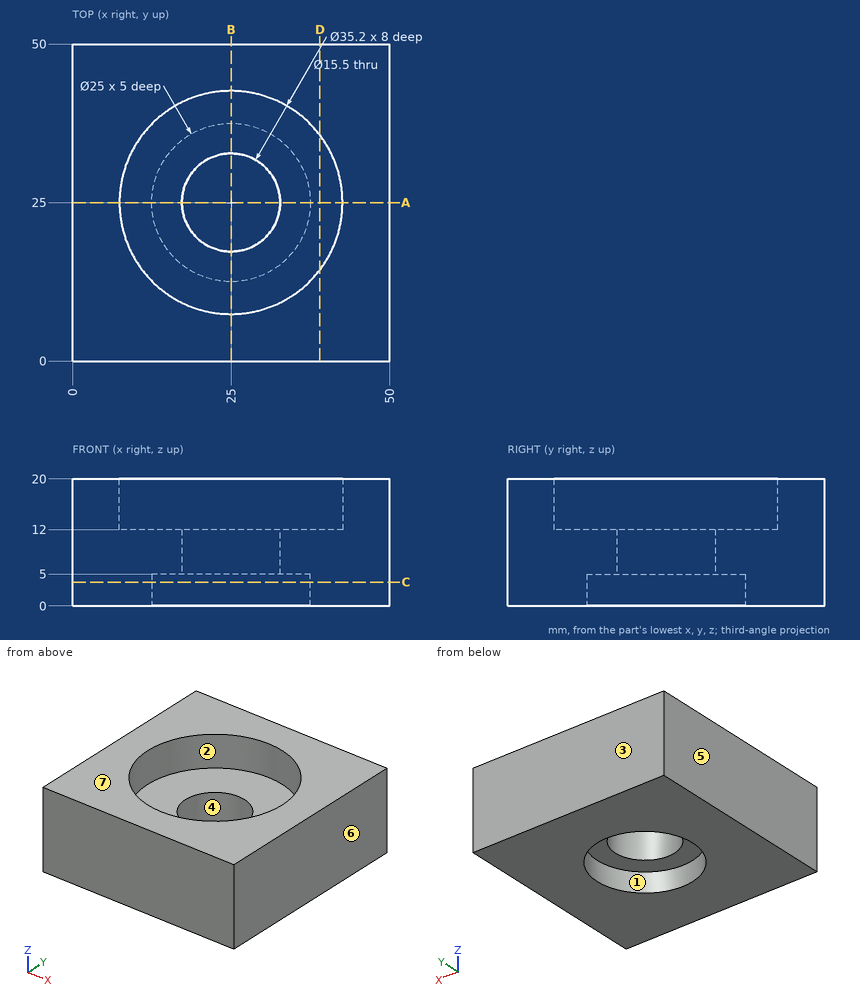
Answer from the drawing. Dimensions are ordinates in mm from the lowest x, y and z of the part. A direction names the side the tool comes from. Give positions to 0.01 mm unless a question says otherwise; leave off trailing zeros. Loops run counter-clockwise (first coordinate to the right, second up) from the corner with the lowest first, then second, coordinate; pieces in that order, holes last. Notation, with made-up numbers: (19, -30.5) -> (66, -30.5) arc R9 cw to (66, -22.5) -> close; hole circle Ø10 at (21, 6.5). An arc over 180 degrees is marked (long way). One line per question, with ' | ' between items. Start each with the question number.
1) Section A-A, the plane y = 25 is taken. Determine the outline of the cut face in (x, z), then the cut area to 3 significant figures.
2) Straight lines are drawn through the part: L1, parallel to Y at x = 25, z = 16; L2, parallel to Y at x = 25, z = 2.9; L3, parallel to Z at x = 36, y = 14. For each, find the intervals that lie inside material, in ascending order.
3) For the marked faces 1, 2 and 3, determine the directions among +Z, -Z, +X, -X, +Y, -Y from which every point of the face is accessible in a straight line to the end or side of a thin tool.
4) Each of these flat-tipped pins is pushed along its axis until it touches: pin 1 (21 mm diameter, centred on x = 25, y = 25, fed in from -Z); pin 2 (25 mm diameter, centred on x = 25, y = 25, fed in from +Z). Where does it stop, or does it pass through?
5) Section D-D, the plane x = 39 is taken. Determine the outline of the cut face in (y, z), then the cut area to 3 significant figures.
6) Section C-C, the plane z = 3.75 is taken. Determine the outline of the cut face in (x, y).
7) Determine the mould class of the marked faces 4, 5, 6 and 7 for opening direction X: +X half, -X half, draft (parallel to the pull), parting line (faces both ways), or undercut.
Resolved:
1) outline: (0, 0) -> (12.5, 0) -> (12.5, 5) -> (17.25, 5) -> (17.25, 12) -> (7.4, 12) -> (7.4, 20) -> (0, 20) -> close; (32.75, 5) -> (37.5, 5) -> (37.5, 0) -> (50, 0) -> (50, 20) -> (42.6, 20) -> (42.6, 12) -> (32.75, 12) -> close | area: 485 mm2
2) L1: 0 to 7.4, 42.6 to 50 | L2: 0 to 12.5, 37.5 to 50 | L3: 0 to 12
3) face 1: -Z | face 2: +Z | face 3: +Z, -Z, +X, -X, +Y
4) pin 1: z = 5 | pin 2: z = 12
5) outline: (0, 0) -> (50, 0) -> (50, 20) -> (35.67, 20) -> (35.67, 12) -> (14.33, 12) -> (14.33, 20) -> (0, 20) -> close | area: 829 mm2
6) outline: (0, 0) -> (50, 0) -> (50, 50) -> (0, 50) -> close; hole circle Ø25 at (25, 25)
7) face 4: undercut | face 5: -X half | face 6: +X half | face 7: draft
